from build123d import *

# Parameters (mm, degrees)
ESBO_O2_R                = 1.5
ESBO_O2_R_2              = 3.425
RESSALTO_EXTRUS_O1_DEPTH = 4.15


with BuildPart() as part:
    # Esboço2 → Ressalto-extrusão1 (new body)
    with BuildSketch(Plane.XY):
        with BuildLine():
            Line((0, 0), (23.7, 0))
            ThreePointArc((23.7, 0), (30.771067812, 2.928932188), (33.7, 10))
            Line((33.7, 10), (33.7, 15))
            ThreePointArc((33.7, 15), (36.628932188, 22.071067812), (43.7, 25))
            Line((43.7, 25), (81.1, 25))
            ThreePointArc((81.1, 25), (88.171067812, 22.071067812), (91.1, 15))
            Line((91.1, 15), (91.1, 10))
            ThreePointArc((91.1, 10), (94.028932188, 2.928932188), (101.1, 0))
            Line((101.1, 0), (124.8, 0))
            Line((124.8, 0), (124.8, 38.959077337))
            ThreePointArc((124.8, 38.959077337), (123.353473382, 43.22040734), (119.611733316, 45.720558121))
            Line((119.611733316, 45.720558121), (86.1, 54.7))
            ThreePointArc((86.1, 54.7), (78.117314341, 116.973565182), (75.45, 179.7))
            Line((75.45, 179.7), (49.35, 179.7))
            ThreePointArc((49.35, 179.7), (46.682685659, 116.973565182), (38.7, 54.7))
            Line((38.7, 54.7), (5.188266684, 45.720558121))
            ThreePointArc((5.188266684, 45.720558121), (1.446526618, 43.22040734), (0, 38.959077337))
            Line((0, 38.959077337), (0, 0))
        make_face()
        with Locations(Location((62.4, 159.5, 0), (0, 0, 180))):
            Circle(ESBO_O2_R, mode=Mode.SUBTRACT)
        with Locations(Location((54.4, 133.5, 0), (0, 0, 180))):
            Circle(ESBO_O2_R, mode=Mode.SUBTRACT)
        with Locations(Location((70.4, 133.5, 0), (0, 0, 180))):
            Circle(ESBO_O2_R, mode=Mode.SUBTRACT)
        with Locations(Location((62.4, 98.575, 0), (0, 0, 180))):
            Circle(ESBO_O2_R_2, mode=Mode.SUBTRACT)
        with Locations(Location((66.3, 77.1, 0), (0, 0, 180))):
            Circle(ESBO_O2_R, mode=Mode.SUBTRACT)
        with Locations(Location((66.3, 44.1, 0), (0, 0, 180))):
            Circle(ESBO_O2_R, mode=Mode.SUBTRACT)
        with Locations(Location((103.9, 36.5, 0), (0, 0, 180))):
            Circle(ESBO_O2_R, mode=Mode.SUBTRACT)
        with Locations(Location((20.9, 36.5, 0), (0, 0, 180))):
            Circle(ESBO_O2_R, mode=Mode.SUBTRACT)
    extrude(amount=RESSALTO_EXTRUS_O1_DEPTH)


solid = part.part
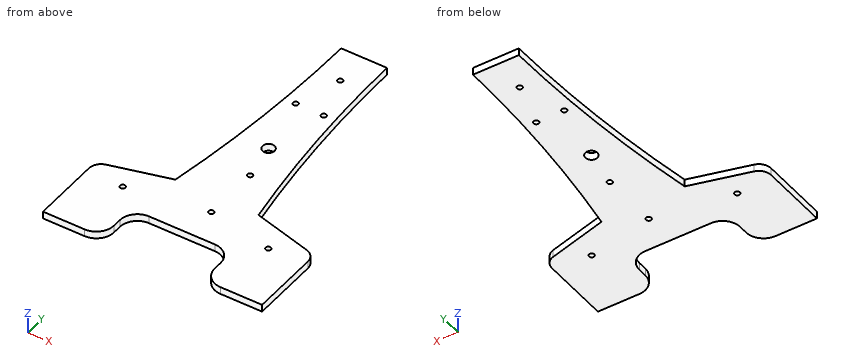
The listing builds one solid part. Answer for the finished solid, in the listing's coordinates (mm). Coordinates: 2 decimals unless noted, no trailing zeros. Order: outer loops, then holes, each group sorted by start corner. A loop starts at its lowest first (then second) coordinate and runs counter-clockwise, first axis right, second up. Notation, with made-up numbers: M 10,-25 L 26,-25 A32 cw 26,3 Z; hole C 52.25,20 d8. An arc over 180 degrees is marked long. Use CSV: the item, a comma, the result in double quotes.
Q1. Section C-C (x = 41.5) is taken. Determine the outline of the cut face in (y, z) (3 decimals), then the cut area to 3 significant figures.
Here are the results:
outline,"M 24.755,0 L 72.28,0 L 72.28,4.15 L 24.755,4.15 Z"
area,"197 mm2"
Q2. Straight lines are drawn through the part: L1, parallel to Y at x = 62.4, z = 2.4; L2, parallel to X at y = 36.5, z = 2.95; L3, parallel to Y at x = 66.3, z = 2.4. For each, find the intervals that lie inside material, in ascending order.
Here are the results:
L1,"25 to 95.15, 102 to 158, 161 to 179.7"
L2,"0 to 19.4, 22.4 to 102.4, 105.4 to 124.8"
L3,"25 to 42.6, 45.6 to 75.6, 78.6 to 179.7"
Q3. Section B-B (y = 164.5) is taken. Determine the outline of the cut face in (x, z).
Here are the results:
outline,"M 49.19,0 L 75.61,0 L 75.61,4.15 L 49.19,4.15 Z"
Q4. Section A-A (z = 0.8) is taken. Give the number of separate pieces and of enclosed holes in the cut face, then the cut area to 3 significant figures.
Here are the results:
separate pieces,"1"
enclosed holes,"8"
area,"9,040 mm2"
Q5. Given pin 1 Ø1.5 at (x, z) = (61, 2.5) entering from -Y; pin 2 Ø1.8 at (x, y) = (103.9, 36.5) entering from +Z; pin 3 Ø4 at (x, y) = (62.4, 159.5) entering from +Z, each flat-ended and moving along its own axis, determine where each tip first touches the part or whether it passes through.
Here are the results:
pin 1,"y = 25"
pin 2,"through"
pin 3,"z = 4.15"
